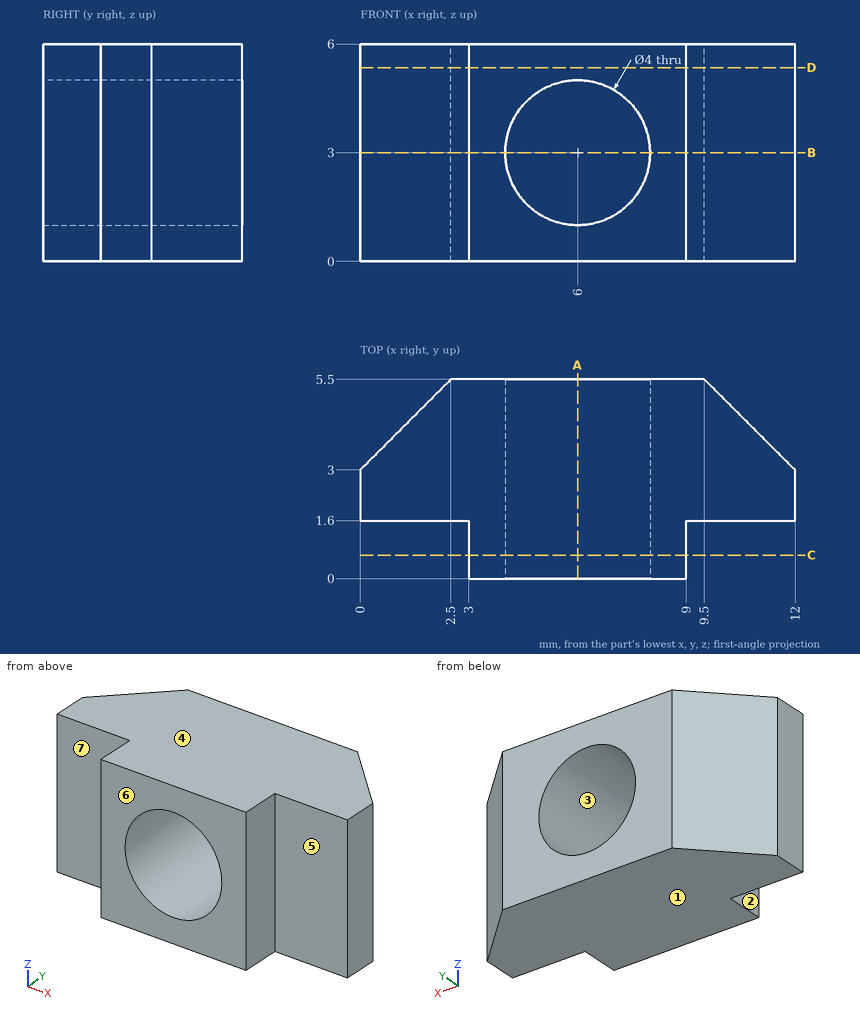
Study the drawing (mm; zero at the part's minimum x, y, z) and answer. A direction names the side the tool comes from. Round coordinates to 2 decimals unless told otherwise and drop trailing zeros. Order: outer loops, then holes, each group sorted by start corner. A loop starts at its lowest first (then second) coordinate and runs counter-clockwise, first axis right, second up. Notation, with made-up numbers: (52.25, 42) -> (94.25, 42) arc R26 ccw to (94.25, 67) -> close; hole circle Ø11 at (-31.5, 76). An arc over 180 degrees is marked (long way). Answer as CSV lines item,"result". Start each with the question number.
(1) The part is cut by section C-C (y = 0.65). Determine the outline of the cut face in (x, z).
(2) Find the intervals of material crossed by probe 1 along Z at (x, y) = (6, 4.1); probe 2 along X at (y, z) = (1.55, 3); probe 3 along X at (y, z) = (1.7, 2.3), in increasing order. Write a range as from..to.
(3) Flat-ended cylindrical pins translate along their axes: pin 1 Ø1.8 at (y, z) = (0.5, 3) entering from -X; pin 2 Ø3 at (x, z) = (6, 3) entering from -Y; pin 3 Ø0.9 at (x, z) = (10.5, 3) entering from -Y. Find the tip coordinate at first contact, or state that the pin passes through.
(4) The part is cut by section B-B (z = 3). Determine the outline of the cut face in (x, y), then the cut area to 4 significant figures.
(5) A tool of negligible diameter and unlimited length cuts with its end or side. For the marked faces 5, 6 and 7, from which of +Z, -Z, +X, -X, +Y, -Y can it reach the whole face along a straight path? Write none if from no direction.
(6) The part is cut by section A-A (x = 6). Determine the outline of the cut face in (y, z), then the cut area to 3 significant figures.
(7) For a pull along Z with two mould halves and no side action, classify the marked faces 1, 2, 3 and 4 as +Z half, -Z half, draft (parallel to the pull), parting line (faces both ways), or undercut.
(8) The part is cut by section D-D (z = 5.35). Determine the outline of the cut face in (x, y).
Evaluation:
1,outline,"(3, 0) -> (9, 0) -> (9, 6) -> (3, 6) -> close; hole circle Ø4 at (6, 3)"
2,probe 1,"0..1, 5..6"
2,probe 2,"3..4, 8..9"
2,probe 3,"0..4.13, 7.87..12"
3,pin 1,"x = 3"
3,pin 2,"through"
3,pin 3,"y = 1.6"
4,outline,"(0, 1.6) -> (3, 1.6) -> (3, 0) -> (4, 0) -> (4, 5.5) -> (2.5, 5.5) -> (0, 3) -> close; (8, 0) -> (9, 0) -> (9, 1.6) -> (12, 1.6) -> (12, 3) -> (9.5, 5.5) -> (8, 5.5) -> close"
4,area,"28.15 mm²"
5,face 5,"+Z, -Z, +X, -Y"
5,face 6,"+Z, -Z, +X, -X, -Y"
5,face 7,"+Z, -Z, -X, -Y"
6,outline,"(0, 0) -> (5.5, 0) -> (5.5, 1) -> (0, 1) -> close; (0, 5) -> (5.5, 5) -> (5.5, 6) -> (0, 6) -> close"
6,area,"11.0 mm²"
7,face 1,"-Z half"
7,face 2,"draft"
7,face 3,"undercut"
7,face 4,"+Z half"
8,outline,"(0, 1.6) -> (3, 1.6) -> (3, 0) -> (9, 0) -> (9, 1.6) -> (12, 1.6) -> (12, 3) -> (9.5, 5.5) -> (2.5, 5.5) -> (0, 3) -> close"
